from build123d import *

# Parameters (mm, degrees)
SKETCH1_W             = 8
SKETCH1_H             = 8
BOSS_EXTRUDE1_DEPTH   = 3
BODY_MOVE_COPY1_ANGLE = 90


with BuildPart() as part:
    # Sketch1 → Loft1 section 0
    with BuildSketch(Plane(origin=(0, 0, 0), x_dir=(1, 0, 0), z_dir=(0, 1, 0)), mode=Mode.PRIVATE) as loft1_s0:
        Rectangle(SKETCH1_W, SKETCH1_H)
    loft([Vertex(0, 8, 0), loft1_s0.sketch])


with BuildPart() as body_2:
    # Sketch5 → Boss-Extrude1 (new body)
    with BuildSketch(Plane.XY):
        Polygon((0, 6), (-2, 2), (2, 2), align=None)
    extrude(amount=BOSS_EXTRUDE1_DEPTH)


with BuildPart() as body_3:
    # Body-Move/Copy1: copy of body 2
    add(body_2.part.rotate(Axis((0, 0, 0), (0, 1, 0)), BODY_MOVE_COPY1_ANGLE))


with BuildPart() as part_1:
    add(part.part)

    # Combine1: union body 2, body 3
    add(body_2.part)
    add(body_3.part)


solid = part_1.part
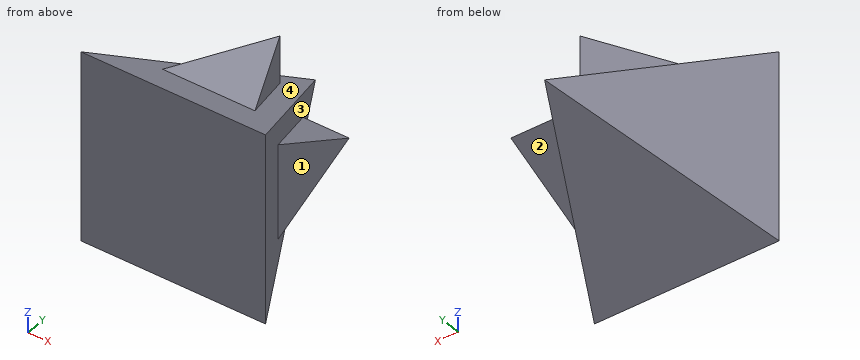
Input: part model. Units: mm. Frame: model coordinates. Face numbers are marked on the shaded views. A direction names the side the tool comes from. Round coordinates to 2 decimals unless told otherwise and drop trailing zeros. Order: outer loops, then holes, each group sorted by start corner. A loop starts at its lowest first (then second) coordinate and runs counter-clockwise, first axis right, second up. Notation, with made-up numbers: (41, 77) - (100, 77) arc R37 ccw to (100, 113) - close; hole circle Ø8 at (-23, 56.25). An arc over 180 degrees is marked (long way). Use a Markdown table: item, result.
1. Section A-A on z = 0.75. Return the cut outline in (x, y), then the cut area to 3 significant figures.
Evaluation:
| item | result |
|---|---|
| outline | (-4, 0) - (4, 0) - (3, 2) - (3, 4.5) - (1.75, 4.5) - (0.75, 6.5) - (-0.75, 6.5) - close |
| area | 32.4 mm^2 |
2. Section C-C on x = 0.75. Return the cut outline in (y, z), then the cut area to 3 significant figures.
Evaluation:
| item | result |
|---|---|
| outline | (0, -4) - (6.5, -0.75) - (6.5, 0.75) - (4.5, 1.75) - (4.5, 3) - (2, 3) - (0, 4) - close |
| area | 32.4 mm^2 |
3. Section D-D on y = 5. Return the cut outline in (x, z), then the cut area to 3 significant figures.
Evaluation:
| item | result |
|---|---|
| outline | (-1.5, -1.5) - (1.5, -1.5) - (1.5, -0.5) - (3, -0.5) - (3, 0.5) - (1.5, 0.5) - (1.5, 1.5) - (0.5, 1.5) - (0.5, 3) - (-0.5, 3) - (-0.5, 1.5) - (-1.5, 1.5) - close |
| area | 12.0 mm^2 |
4. Material intervals for probe 1 along Y at (x, z) = (-3.5, -3.25); probe 2 along Y at (x, z) = (-0.75, 1); probe 3 along Z at (x, y) = (1.25, 5.75) (3 decimals), sorted ascending.
Evaluation:
| item | result |
|---|---|
| probe 1 | 0 to 1 |
| probe 2 | 0 to 6 |
| probe 3 | -0.125 to 0.125 |
5. Section B-B on y = 4. Return the cut outline in (x, z), then the cut area to 3 significant figures.
Evaluation:
| item | result |
|---|---|
| outline | (-2, -2) - (2, -2) - (2, -1) - (3, -1) - (3, 1) - (2, 1) - (2, 2) - (1, 2) - (1, 3) - (-1, 3) - (-1, 2) - (-2, 2) - close |
| area | 20.0 mm^2 |
6. First-contact query: pin 1 (3 mm diameter, centred on y = 5, z = 1, fed in from +X); pin 2 (1.5 mm diameter, centred on x = -0.5, z = 0.5, fed in from -Y); pin 3 (1.2 mm diameter, centred on x = 0.5, y = 3, fed in from +Z); pin 4 (1.5 mm diameter, centred on x = 0, z = 1.5, fed in from +Y). Flat tips, straight axial feed; report the tip coordinate or a pass-through.
Evaluation:
| item | result |
|---|---|
| pin 1 | x = 3 |
| pin 2 | y = 0 |
| pin 3 | z = 3 |
| pin 4 | y = 6.5 |
7. Access query for the marked faces 1, 2, 3 and 4. Directions: +Z, -Z, +X, -X, +Y, -Y. A direction counts if a zero-diameter tool reaches every point of the face in a straight line with its end or side. Return the directions, or none.
Evaluation:
| item | result |
|---|---|
| face 1 | +Z, -Z, +X, +Y |
| face 2 | -Z, +X, +Y |
| face 3 | +X, +Y |
| face 4 | +Z, +Y |
